Part model, mm, in its own coordinate system. Round coordinates to 2 decimals unless told otherwise and drop trailing zeros. Loops run counter-clockwise (first coordinate to the right, second up) from the corner with the lowest first, then second, coordinate; pieces in that order, holes last. Notation, with made-up numbers: M 47.5,11.5 L 62.5,11.5 A21 ccw 62.5,45.5 Z; hole C 14.25,54 d6. An arc over 180 degrees is marked long. Put each result on its own line as item: value. Start each with the question number.
```python
from build123d import *

# Parameters (mm, degrees)
SKETCH_1_R      = 1.75
EXTRUDE_3_DEPTH = 2
EXTRUDE_3_DRAFT = -1
EXTRUDE_4_DEPTH = 22


with BuildPart() as part:
    # 草图1 → 凸台-拉伸3 (with draft: the straight prism first)
    with BuildSketch(Plane.XY):
        with BuildLine():
            ThreePointArc((0, 2.744628665), (0.803883124, 0.803883124), (2.744628665, 0))
            Line((2.744628665, 0), (97.255371335, 0))
            ThreePointArc((97.255371335, 0), (99.196116876, 0.803883124), (100, 2.744628665))
            Line((100, 2.744628665), (100, 36.255371335))
            ThreePointArc((100, 36.255371335), (99.196116876, 38.196116876), (97.255371335, 39))
            Line((97.255371335, 39), (79, 39))
            Line((79, 39), (79, 20.25))
            Line((79, 20.25), (21, 20.25))
            Line((21, 20.25), (21, 39))
            Line((21, 39), (2.744628665, 39))
            ThreePointArc((2.744628665, 39), (0.803883124, 38.196116876), (0, 36.255371335))
            Line((0, 36.255371335), (0, 2.744628665))
        make_face()
        with BuildLine():
            ThreePointArc((11.25, 6.25), (8, 3), (4.75, 6.25))
            Line((4.75, 6.25), (4.75, 13.75))
            ThreePointArc((4.75, 13.75), (8, 17), (11.25, 13.75))
            Line((11.25, 13.75), (11.25, 6.25))
        make_face(mode=Mode.SUBTRACT)
        with BuildLine():
            ThreePointArc((25.25, 6.25), (22, 3), (18.75, 6.25))
            Line((18.75, 6.25), (18.75, 13.75))
            ThreePointArc((18.75, 13.75), (22, 17), (25.25, 13.75))
            Line((25.25, 13.75), (25.25, 6.25))
        make_face(mode=Mode.SUBTRACT)
        with BuildLine():
            ThreePointArc((39.25, 6.25), (36, 3), (32.75, 6.25))
            Line((32.75, 6.25), (32.75, 13.75))
            ThreePointArc((32.75, 13.75), (36, 17), (39.25, 13.75))
            Line((39.25, 13.75), (39.25, 6.25))
        make_face(mode=Mode.SUBTRACT)
        with BuildLine():
            ThreePointArc((53.25, 6.25), (50, 3), (46.75, 6.25))
            Line((46.75, 6.25), (46.75, 13.75))
            ThreePointArc((46.75, 13.75), (50, 17), (53.25, 13.75))
            Line((53.25, 13.75), (53.25, 6.25))
        make_face(mode=Mode.SUBTRACT)
        with BuildLine():
            ThreePointArc((67.25, 6.25), (64, 3), (60.75, 6.25))
            Line((60.75, 6.25), (60.75, 13.75))
            ThreePointArc((60.75, 13.75), (64, 17), (67.25, 13.75))
            Line((67.25, 13.75), (67.25, 6.25))
        make_face(mode=Mode.SUBTRACT)
        with BuildLine():
            ThreePointArc((81.25, 6.25), (78, 3), (74.75, 6.25))
            Line((74.75, 6.25), (74.75, 13.75))
            ThreePointArc((74.75, 13.75), (78, 17), (81.25, 13.75))
            Line((81.25, 13.75), (81.25, 6.25))
        make_face(mode=Mode.SUBTRACT)
        with BuildLine():
            ThreePointArc((95.25, 6.25), (92, 3), (88.75, 6.25))
            Line((88.75, 6.25), (88.75, 13.75))
            ThreePointArc((88.75, 13.75), (92, 17), (95.25, 13.75))
            Line((95.25, 13.75), (95.25, 6.25))
        make_face(mode=Mode.SUBTRACT)
        with Locations((15, 29)):
            Circle(SKETCH_1_R, mode=Mode.SUBTRACT)
        with Locations((85, 29)):
            Circle(SKETCH_1_R, mode=Mode.SUBTRACT)
        with Locations((15, 36)):
            Circle(SKETCH_1_R, mode=Mode.SUBTRACT)
        with Locations((85, 36)):
            Circle(SKETCH_1_R, mode=Mode.SUBTRACT)
    extrude(amount=EXTRUDE_3_DEPTH)
    # 凸台-拉伸3: the draft: its side faces are tilted about the plane it starts from
    extrude_3_sides = [part.faces().sort_by_distance(p)[0] for p in [
        (21, 29.625, 1),
        (11.872314333, 39, 1),
        (0.803883124, 38.196116876, 1),
        (0, 19.5, 1),
        (0.803883124, 0.803883124, 1),
        (50, 0, 1),
        (99.196116876, 0.803883124, 1),
        (100, 19.5, 1),
        (99.196116876, 38.196116876, 1),
        (88.127685667, 39, 1),
        (79, 29.625, 1),
        (50, 20.25, 1),
        (4.75, 10, 1),
        (8, 17, 1),
        (11.25, 10, 1),
        (8, 3, 1),
        (22, 17, 1),
        (25.25, 10, 1),
        (22, 3, 1),
        (18.75, 10, 1),
        (32.75, 10, 1),
        (36, 17, 1),
        (39.25, 10, 1),
        (36, 3, 1),
        (50, 3, 1),
        (46.75, 10, 1),
        (50, 17, 1),
        (53.25, 10, 1),
        (64, 17, 1),
        (67.25, 10, 1),
        (64, 3, 1),
        (60.75, 10, 1),
        (78, 17, 1),
        (81.25, 10, 1),
        (78, 3, 1),
        (74.75, 10, 1),
        (92, 17, 1),
        (95.25, 10, 1),
        (92, 3, 1),
        (88.75, 10, 1),
        (13.25, 29, 1),
        (83.25, 29, 1),
        (13.25, 36, 1),
        (83.25, 36, 1),
    ]]
    draft(extrude_3_sides, Plane.XY, EXTRUDE_3_DRAFT)

    # 草图1<8> → 凸台-拉伸4 (add)
    with BuildSketch(Plane.XY):
        with BuildLine():
            ThreePointArc((0, 2.744628665), (0.803883124, 0.803883124), (2.744628665, 0))
            Line((2.744628665, 0), (97.255371335, 0))
            ThreePointArc((97.255371335, 0), (99.196116876, 0.803883124), (100, 2.744628665))
            Line((100, 2.744628665), (100, 20.25))
            Line((100, 20.25), (79, 20.25))
            Line((79, 20.25), (21, 20.25))
            Line((21, 20.25), (0, 20.25))
            Line((0, 20.25), (0, 2.744628665))
        make_face()
        with BuildLine():
            ThreePointArc((11.25, 6.25), (8, 3), (4.75, 6.25))
            Line((4.75, 6.25), (4.75, 13.75))
            ThreePointArc((4.75, 13.75), (8, 17), (11.25, 13.75))
            Line((11.25, 13.75), (11.25, 6.25))
        make_face(mode=Mode.SUBTRACT)
        with BuildLine():
            ThreePointArc((25.25, 6.25), (22, 3), (18.75, 6.25))
            Line((18.75, 6.25), (18.75, 13.75))
            ThreePointArc((18.75, 13.75), (22, 17), (25.25, 13.75))
            Line((25.25, 13.75), (25.25, 6.25))
        make_face(mode=Mode.SUBTRACT)
        with BuildLine():
            ThreePointArc((39.25, 6.25), (36, 3), (32.75, 6.25))
            Line((32.75, 6.25), (32.75, 13.75))
            ThreePointArc((32.75, 13.75), (36, 17), (39.25, 13.75))
            Line((39.25, 13.75), (39.25, 6.25))
        make_face(mode=Mode.SUBTRACT)
        with BuildLine():
            ThreePointArc((53.25, 6.25), (50, 3), (46.75, 6.25))
            Line((46.75, 6.25), (46.75, 13.75))
            ThreePointArc((46.75, 13.75), (50, 17), (53.25, 13.75))
            Line((53.25, 13.75), (53.25, 6.25))
        make_face(mode=Mode.SUBTRACT)
        with BuildLine():
            ThreePointArc((67.25, 6.25), (64, 3), (60.75, 6.25))
            Line((60.75, 6.25), (60.75, 13.75))
            ThreePointArc((60.75, 13.75), (64, 17), (67.25, 13.75))
            Line((67.25, 13.75), (67.25, 6.25))
        make_face(mode=Mode.SUBTRACT)
        with BuildLine():
            ThreePointArc((81.25, 6.25), (78, 3), (74.75, 6.25))
            Line((74.75, 6.25), (74.75, 13.75))
            ThreePointArc((74.75, 13.75), (78, 17), (81.25, 13.75))
            Line((81.25, 13.75), (81.25, 6.25))
        make_face(mode=Mode.SUBTRACT)
        with BuildLine():
            ThreePointArc((95.25, 6.25), (92, 3), (88.75, 6.25))
            Line((88.75, 6.25), (88.75, 13.75))
            ThreePointArc((88.75, 13.75), (92, 17), (95.25, 13.75))
            Line((95.25, 13.75), (95.25, 6.25))
        make_face(mode=Mode.SUBTRACT)
    extrude(amount=EXTRUDE_4_DEPTH)


solid = part.part
```
1. Cut at B-B, the plane z = 9.25. Give the number of separate pieces and of enclosed holes in the cut face, and give its area (3 significant figures).
2. Wall check: L1, parallel to Y at x = 78, z = 11; L2, parallel to Y at x = 28, z = 11.25; L3, parallel to Z at x = 14, y = 21. Give the ranges that are in metal, low to high.
3. Drop flat-ended pins along their axis: pin 1 (2 mm diameter, centred on y = 11.5, z = 16, fed in from -X); pin 2 (3 mm diameter, centred on x = 35, y = 9.5, fed in from +Z); pin 3 (5 mm diameter, centred on y = 15, z = 11.5, fed in from +X); pin 4 (2 mm diameter, centred on x = 45.5, z = 5, fed in from +Y). Give the stop position or say it passes through.
4. Cut at A-A, the plane y = 25. Give the cut face in (x, z).
5. Mould opens along X. For faces 1 (the conical face through (50.07, 3.02, 0.99)), 2 (the flat face through (0, 12, 12)) say: released by +X, released by -X, zero draft, split by the parting line, or undercut.
Results list:
1. separate pieces: 1
1. enclosed holes: 7
1. area: 1,450 mm^2
2. L1: y = 0 to 3, 17 to 20.25
2. L2: y = 0 to 20.25
2. L3: z = 0 to 2
3. pin 1: stops at x = 0
3. pin 2: passes through
3. pin 3: stops at x = 100
3. pin 4: stops at y = 20.25
4. outline: M -0.03,2 L 0,0 L 21,0 L 21.03,2 Z; M 78.97,2 L 79,0 L 100,0 L 100.03,2 Z
5. face 1: undercut
5. face 2: released by -X
